Work out the finished part from the listing and answer in its coordinate system (mm). Round coordinates to 2 decimals unless told otherwise and drop trailing zeros. Order: outer loops, then holes, each group sorted by start corner. A loop starts at its lowest first (then second) coordinate and runs counter-clockwise, first axis right, second up. Notation, with made-up numbers: (34, 26) - (86, 26) arc R9 ccw to (86, 39) - close; hole circle Ø3 at (34.25, 79). An arc over 180 degrees is marked (long way). Answer in a Markdown table with one row per item.
from build123d import *


with BuildPart() as part:
    # Sketch1 → Revolve1 (revolve)
    with BuildSketch(Plane(origin=(0, 0, 0), x_dir=(0, 0, -1), z_dir=(1, 0, 0)), mode=Mode.PRIVATE) as revolve1_sk:
        with BuildLine():
            Line((0, 1.5), (2, 1.5))
            Line((2, 1.5), (2, 3))
            ThreePointArc((2, 3), (2.643776387, 2.065664221), (3.033380227, 1))
            Line((3.033380227, 1), (2.833380227, 1))
            Line((2.833380227, 1), (2.833380227, 0))
            Line((2.833380227, 0), (-3.355203179, 0))
            ThreePointArc((-3.355203179, 0), (-3.014528985, 0.822460259), (-2.192068726, 1.163134453))
            ThreePointArc((-2.192068726, 1.163134453), (-1.18922755, 1.937998702), (0, 1.5))
        make_face()
    revolve(revolve1_sk.sketch.rotate(Axis((0, 0, -2.612732095), (0, 0, 1)), 90), axis=Axis((0, 0, -2.612732095), (0, 0, 1)))


solid = part.part
1) Each of these flat-tipped pins is pushed along its axis until it touches: pin 1 (2 mm diameter, centred on x = 2.5, z = 1, fed in from +Y); pin 2 (1 mm diameter, centred on y = 1, z = 2, fed in from -X); pin 3 (1 mm diameter, centred on x = 0, y = 0, fed in from -Z). Where does it stop, or does it pass through?
Filled in:
| item | result |
|---|---|
| pin 1 | stops at y = 1.25 |
| pin 2 | stops at x = -1.66 |
| pin 3 | stops at z = -2.83 |
2) Find section D-D, the plane z = 3. Give the vertices of the cut face in (x, y).
Filled in:
| item | result |
|---|---|
| outline | circle Ø1.67 at (0, 0) |
3) Find section A-A, the plane y = -2.55. Give the vertices of the cut face in (x, z).
Filled in:
| item | result |
|---|---|
| outline | (-1.58, -2) arc R3.71 ccw to (1.58, -2) - close |
4) The mould has two halves that part along Y. Classify faces 1 (the face through (0, 0, -2.833)), 2 (the face through (-1.43, -0.45, -1.01)), 3 (the face through (1.3, 1.3, -2)): released by +Y, released by -Y, zero draft, split by the parting line, or undercut.
Filled in:
| item | result |
|---|---|
| face 1 | undercut |
| face 2 | split by the parting line |
| face 3 | zero draft |
5) Find the intervals of material crossed by probe 1 along Z at (x, y) = (2.45, -1.4); probe 2 along X at (y, z) = (0.6, 1); probe 3 along X at (y, z) = (-0.75, 1.5), in increasing order. Write a range as from..to.
Filled in:
| item | result |
|---|---|
| probe 1 | z = -2.15..-2 |
| probe 2 | x = -1.86..1.86 |
| probe 3 | x = -1.69..1.69 |
6) Find section B-B, the plane z = -2.5. Give the vertices of the cut face in (x, y), then the cut area to 3 significant figures.
Filled in:
| item | result |
|---|---|
| outline | circle Ø4.65 at (0, 0) |
| area | 17.0 mm^2 |
